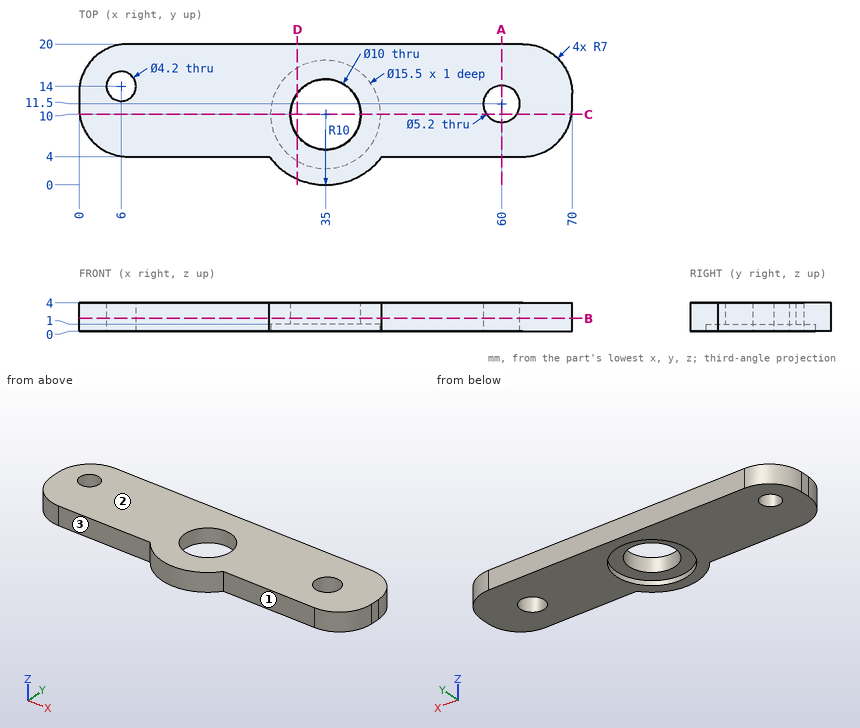
Can you work these out from the drawing? Everything is in mm from the part's minimum corner. A direction names the side the tool comes from. Round coordinates to 2 decimals unless told otherwise and drop trailing zeros. Loops run counter-clockwise (first coordinate to the right, second up) from the corner with the lowest first, then second, coordinate; pieces in that order, holes last. Notation, with made-up numbers: (51, 76) -> (98, 76) arc R21 ccw to (98, 111) -> close; hole circle Ø3 at (76.25, 70.5). An arc over 180 degrees is marked (long way). Use CSV: the item, a comma, the result in double quotes.
(1) Suppose I cut it at B-B on z = 1.8. Write out the boundary of the cut face in (x, y), plus the area to 3 significant figures.
Return value:
outline,"(0, 11) arc R7 ccw to (7, 4) -> (27, 4) arc R10 ccw to (43, 4) -> (63, 4) arc R7 ccw to (70, 11) -> (70, 13) arc R7 ccw to (63, 20) -> (7, 20) arc R7 ccw to (0, 13) -> close; hole circle Ø4.2 at (6, 14); hole circle Ø10 at (35, 10); hole circle Ø5.2 at (60, 11.5)"
area,"1,010 mm²"
(2) Suppose I cut it at A-A on x = 60. Write out the boundary of the cut face in (y, z).
Return value:
outline,"(4, 0) -> (8.9, 0) -> (8.9, 4) -> (4, 4) -> close; (14.1, 0) -> (20, 0) -> (20, 4) -> (14.1, 4) -> close"
(3) For the marked faces 1, 2 and 3, which set-ups out of +Z, -Z, +X, -X, +Y, -Y let a thin tool reach every point of the face, with its end or its side?
Return value:
face 1,"+Z, -Z, +X, -Y"
face 2,"+Z, +X, -X, +Y, -Y"
face 3,"+Z, -Z, -X, -Y"
(4) If I drill on probe 1 along Y at (x, z) = (35, 0.7); probe 2 along X at (y, z) = (9.5, 2.2); probe 3 along Y at (x, z) = (35, 2.25), over which ranges is the centre line in solid material (lowest first)? Write a range as [from, to].
Return value:
probe 1,"y = [0, 2.25], [17.75, 20]"
probe 2,"x = [0.16, 30.03], [39.97, 58.34], [61.66, 69.84]"
probe 3,"y = [0, 5], [15, 20]"
(5) Will these pins go through, and if not, where does the flat tip stop? pin 1 Ø3 at (x, y) = (31.5, 5.5) entering from -Z; pin 2 Ø12 at (x, y) = (13, 2.5) entering from -Z; pin 3 Ø1 at (y, z) = (6, 3.5) entering from -X; pin 4 Ø2 at (x, z) = (18.5, 2.5) entering from -Y.
Return value:
pin 1,"stops at z = 1"
pin 2,"stops at z = 0"
pin 3,"stops at x = 1.64"
pin 4,"stops at y = 4"
(6) Suppose I cut it at C-C on y = 10. Write out the boundary of the cut face in (x, z).
Return value:
outline,"(0.07, 0) -> (27.25, 0) -> (27.25, 1) -> (30, 1) -> (30, 4) -> (0.07, 4) -> close; (40, 1) -> (42.75, 1) -> (42.75, 0) -> (57.88, 0) -> (57.88, 4) -> (40, 4) -> close; (62.12, 0) -> (69.93, 0) -> (69.93, 4) -> (62.12, 4) -> close"
(7) Suppose I cut it at D-D on x = 31. Write out the boundary of the cut face in (y, z).
Return value:
outline,"(0.83, 0) -> (3.36, 0) -> (3.36, 1) -> (7, 1) -> (7, 4) -> (0.83, 4) -> close; (13, 1) -> (16.64, 1) -> (16.64, 0) -> (20, 0) -> (20, 4) -> (13, 4) -> close"
